Verification items for the finished model (mm, model axes). Face numbers are marked on the shaded views. A direction names the side the tool comes from. Give positions to 0.01 mm unless a question says otherwise; leave off trailing zeros. Loops run counter-clockwise (first coordinate to the right, second up) from the corner with the lowest first, then second, coordinate; pieces in that order, holes last. Notation, with made-up numbers: (81.5, 3.25) -> (128.5, 3.25) arc R24 cw to (128.5, 25.25) -> close; hole circle Ø10 at (71.25, -12). An arc over 180 degrees is marked (long way). Answer in a Markdown table with one row per item. Add a question column.
Q1. Material ranges on probe 1 along Y at (x, z) = (4, 9.5); probe 2 along X at (y, z) = (-13, 8.25); probe 3 along Z at (x, y) = (31.5, 0.5), recorded low to high.
Q2. Set-up check for the marked faces 1, 2 and 3: record each of +Z, -Z, +X, -X, +Y, -Y from which the full face is reachable in a straight line by a thin tool's end or side.
Q3. Gauge pin test, flat ends, axial feed: P1, Ø4, axis at x = 36.5, y = 18.5, coming from the +Z side; P2, Ø3, axis at x = 65, z = 5.5, coming from the -Y side. Record the tip position at first contact, or that the pin passes through.
Q4. Release check for a two-part mould opening along X. For the marked faces 4, 5, 6 and 7 record: pulls with the +X half, pulls with the -X half, needs draft (parallel to the pull), parting line crosses it, or undercut.
Q5. Section check C-C on z = 4.5. Enter the section's corners in (x, y).
Q6. Section check B-B on y = 22.5. Enter the section's corners in (x, z).
Q7. Section check A-A on x = 7. Enter the section's corners in (y, z).
```python
from build123d import *

# Parameters (mm, degrees)
F0_W         = 99.2175191641
F0_H         = 55.2872437984
F1_DEPTH     = 10
F2_T         = -2.5
F3_R         = 5
F4_T1_DEPTH  = 2.5
F4_S5_W      = 5
F4_S5_H      = 5
F4_T6_DEPTH  = 5
F4_S11_W     = 5
F4_S11_H     = 5
F4_T12_DEPTH = 5
F4_S17_W     = 5
F4_S17_H     = 5
F4_T18_DEPTH = 5
F4_S23_W     = 5
F4_S23_H     = 5
F4_T24_DEPTH = 5
F5_SIZE      = 2
F6_W         = 2.7456413954
F6_H         = 3.2448493876
F6_W_2       = 2.9952451587
F6_H_2       = 3.1200476224
F7_DEPTH     = 58.81103
F8_W         = 30.3268581629
F8_H         = 54.9128409475
F9_DEPTH     = 10.11623


# Not quite as in the source:
# - a fillet or chamfer that OpenCascade refuses, or shapes differently, is made with other operations: its cross-section is extruded or revolved along the edge and cut away or added
# - a feature names something its author has since deleted; it is built from what else it names


with BuildPart() as f1:
    # F0 (on Top) → F1 (new body)
    with BuildSketch(Plane.XY):
        with Locations((6.4272992313, 3.9312606677)):
            Rectangle(F0_W, F0_H)
    extrude(amount=F1_DEPTH)

    # F2
    f2_openings = [f1.faces().sort_by_distance(p)[0] for p in [
        (6.427299, 3.931261, 10),
    ]]
    offset(amount=F2_T, openings=f2_openings)

    # F3
    f3_edges = [f1.edges().sort_by_distance(p)[0] for p in [
        (6.427299, 29.074883, 2.5),
        (-40.68146, 3.931261, 2.5),
        (53.536059, 3.931261, 2.5),
        (6.427299, -21.212361, 2.5),
    ]]
    fillet(f3_edges, radius=F3_R)

    # F4: fillet of radius 5 on 4 edges, made by hand

    # F4_s2 → F4_t1 (join)
    with BuildSketch(Plane.XY.offset(7.5)):
        with BuildLine():
            ThreePointArc((-35.6814603508, 29.0748825669), (-39.2169942567, 27.6104164729), (-40.6814603508, 24.0748825669))
            Line((-40.6814603508, 24.0748825669), (-40.6814603508, 29.0748825669))
            Line((-40.6814603508, 29.0748825669), (-35.6814603508, 29.0748825669))
        make_face()
        with BuildLine():
            ThreePointArc((-40.6814603508, -16.2123612314), (-39.2169942567, -19.7478951374), (-35.6814603508, -21.2123612314))
            Line((-35.6814603508, -21.2123612314), (-40.6814603508, -21.2123612314))
            Line((-40.6814603508, -21.2123612314), (-40.6814603508, -16.2123612314))
        make_face()
        with BuildLine():
            ThreePointArc((53.5360588133, -16.2123612314), (52.0715927193, -19.7478951374), (48.5360588133, -21.2123612314))
            Line((48.5360588133, -21.2123612314), (53.5360588133, -21.2123612314))
            Line((53.5360588133, -21.2123612314), (53.5360588133, -16.2123612314))
        make_face()
        with BuildLine():
            ThreePointArc((48.5360588133, 29.0748825669), (52.0715927193, 27.6104164729), (53.5360588133, 24.0748825669))
            Line((53.5360588133, 24.0748825669), (53.5360588133, 29.0748825669))
            Line((53.5360588133, 29.0748825669), (48.5360588133, 29.0748825669))
        make_face()
    extrude(amount=F4_T1_DEPTH)


with BuildPart() as f4_tool4:
    # F4_s5 → F4_t6 (new body)
    with BuildSketch(Plane.XZ.offset(-24.0748825669)):
        with Locations((51.0360588133, 5)):
            Rectangle(F4_S5_W, F4_S5_H)
    extrude(amount=-F4_T6_DEPTH)

    # F4_s7 → F4_t8 (revolve, cut)
    with BuildSketch(Plane(origin=(48.5360588133, 24.0748825669, 7.5), x_dir=(-0.7071067812, 0, 0.7071067812), z_dir=(-0.7071067812, 0, -0.7071067812))):
        with BuildLine():
            ThreePointArc((0, -5), (5, 0), (0, 5))
            Line((0, 5), (0, -5))
        make_face()
    revolve(axis=Axis((48.5360588133, 24.0748825669, 7.5), (0, 1, 0)), mode=Mode.SUBTRACT)


with BuildPart() as f1_1:
    add(f1.part)

    # F4_t3: union F4_tool4
    add(f4_tool4.part)


with BuildPart() as f4_tool10:
    # F4_s11 → F4_t12 (new body)
    with BuildSketch(Plane.YZ.offset(48.5360588133)):
        with Locations((-18.7123612314, 5)):
            Rectangle(F4_S11_W, F4_S11_H)
    extrude(amount=F4_T12_DEPTH)

    # F4_s13 → F4_t14 (revolve, cut)
    with BuildSketch(Plane(origin=(48.5360588133, -16.2123612314, 7.5), x_dir=(0, 0.7071067812, 0.7071067812), z_dir=(0, 0.7071067812, -0.7071067812))):
        with BuildLine():
            ThreePointArc((0, -5), (5, 0), (0, 5))
            Line((0, 5), (0, -5))
        make_face()
    revolve(axis=Axis((48.5360588133, -16.2123612314, 7.5), (1, 0, 0)), mode=Mode.SUBTRACT)


with BuildPart() as f1_2:
    add(f1_1.part)

    # F4_t9: union F4_tool10
    add(f4_tool10.part)


with BuildPart() as f4_tool16:
    # F4_s17 → F4_t18 (new body)
    with BuildSketch(Plane.YZ.offset(-35.6814603508)):
        with Locations((-18.7123612314, 5)):
            Rectangle(F4_S17_W, F4_S17_H)
    extrude(amount=-F4_T18_DEPTH)

    # F4_s19 → F4_t20 (revolve, cut)
    with BuildSketch(Plane(origin=(-35.6814603508, -16.2123612314, 7.5), x_dir=(0, 0.7071067812, 0.7071067812), z_dir=(0, -0.7071067812, 0.7071067812))):
        with BuildLine():
            ThreePointArc((0, -5), (5, 0), (0, 5))
            Line((0, 5), (0, -5))
        make_face()
    revolve(axis=Axis((-35.6814603508, -16.2123612314, 7.5), (-1, 0, 0)), mode=Mode.SUBTRACT)


with BuildPart() as f1_3:
    add(f1_2.part)

    # F4_t15: union F4_tool16
    add(f4_tool16.part)


with BuildPart() as f4_tool22:
    # F4_s23 → F4_t24 (new body)
    with BuildSketch(Plane.XZ.offset(-24.0748825669)):
        with Locations((-38.1814603508, 5)):
            Rectangle(F4_S23_W, F4_S23_H)
    extrude(amount=-F4_T24_DEPTH)

    # F4_s25 → F4_t26 (revolve, cut)
    with BuildSketch(Plane(origin=(-35.6814603508, 24.0748825669, 7.5), x_dir=(0.7071067812, 0, 0.7071067812), z_dir=(-0.7071067812, 0, 0.7071067812))):
        with BuildLine():
            ThreePointArc((0, -5), (5, 0), (0, 5))
            Line((0, 5), (0, -5))
        make_face()
    revolve(axis=Axis((-35.6814603508, 24.0748825669, 7.5), (0, 1, 0)), mode=Mode.SUBTRACT)


with BuildPart() as f1_4:
    add(f1_3.part)

    # F4_t21: union F4_tool22
    add(f4_tool22.part)

    # F5
    f5_edges = [f1_4.edges().sort_by_distance(p)[0] for p in [
        (56.036059, -23.712361, 5),
        (56.036059, 31.574883, 5),
        (-43.18146, -23.712361, 5),
        (-43.18146, 31.574883, 5),
    ]]
    chamfer(f5_edges, length=F5_SIZE)

    # F6 (on Right) → F7 (cut, symmetric)
    with BuildSketch(Plane.YZ):
        with Locations((-13.6034078896, -0.1248018816)):
            Rectangle(F6_W, F6_H)
        with Locations((19.7187010199, -0.3120047622)):
            Rectangle(F6_W_2, F6_H_2)
    extrude(amount=F7_DEPTH, both=True, mode=Mode.SUBTRACT)

    # F8 (on Top) → F9 (join)
    with BuildSketch(Plane.XY):
        with Locations((68.8282549381, 3.9936611429)):
            Rectangle(F8_W, F8_H)
    extrude(amount=F9_DEPTH)


solid = f1_4.part
```
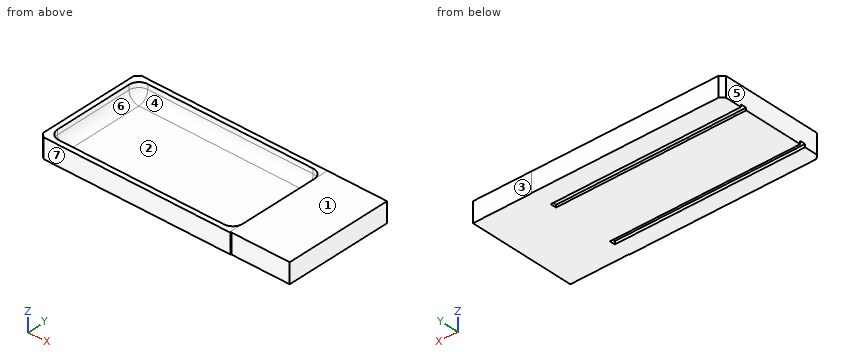
Taken from the geometry:
| question | item | result |
|---|---|---|
| 1 | probe 1 | y = -23.71 to -21.21, 29.07 to 31.57 |
| 1 | probe 2 | x = -43.18 to -40.68, 53.54 to 83.99 |
| 1 | probe 3 | z = 0 to 2.5 |
| 2 | face 1 | +Z, +X, -X, +Y, -Y |
| 2 | face 2 | +Z |
| 2 | face 3 | +Z, -Z, +X, +Y |
| 3 | P1 | stops at z = 2.5 |
| 3 | P2 | stops at y = -23.46 |
| 4 | face 4 | undercut |
| 4 | face 5 | pulls with the -X half |
| 4 | face 6 | undercut |
| 4 | face 7 | needs draft |
| 5 | outline | (-43.18, -21.71) -> (-41.18, -23.71) -> (54.04, -23.71) -> (54.29, -23.46) -> (83.99, -23.46) -> (83.99, 31.45) -> (54.16, 31.45) -> (54.04, 31.57) -> (-41.18, 31.57) -> (-43.18, 29.57) -> close; hole (-39.68, -16.21) arc R4 ccw to (-35.68, -20.21) -> (48.54, -20.21) arc R4 ccw to (52.54, -16.21) -> (52.54, 24.07) arc R4 ccw to (48.54, 28.07) -> (-35.68, 28.07) arc R4 ccw to (-39.68, 24.07) -> close |
| 6 | outline | (-43.18, 0) -> (83.99, 0) -> (83.99, 10.12) -> (53.66, 10.12) -> (53.66, 10) -> (53.54, 10) -> (53.54, 7.5) arc R5 cw to (48.54, 2.5) -> (-35.68, 2.5) arc R5 cw to (-40.68, 7.5) -> (-40.68, 10) -> (-43.18, 10) -> close |
| 7 | outline | (-23.71, 0) -> (-14.98, 0) -> (-14.98, 1.5) -> (-12.23, 1.5) -> (-12.23, 0) -> (18.22, 0) -> (18.22, 1.25) -> (21.22, 1.25) -> (21.22, 0) -> (31.57, 0) -> (31.57, 10) -> (29.07, 10) -> (29.07, 7.5) arc R5 cw to (24.07, 2.5) -> (-16.21, 2.5) arc R5 cw to (-21.21, 7.5) -> (-21.21, 10) -> (-23.71, 10) -> close |
